Here's how the part is built. I have some questions about the finished solid (model axes, mm). Face numbers are marked on the shaded views. A direction names the side the tool comes from. Round coordinates to 2 decimals unless told otherwise and drop trailing zeros. Order: outer loops, then holes, each group sorted by start corner. A loop starts at its lowest first (then second) coordinate and runs counter-clockwise, first axis right, second up. Notation, with made-up numbers: M -14.5,71.5 L -4.5,71.5 A20 ccw -4.5,104.5 Z; hole C 68.25,-12 d3. An arc over 180 degrees is marked long. Answer as CSV lines item,"result". Start each with the question number.
```python
from build123d import *

# Parameters (mm, degrees)
F0_R     = 6.185827
F0_R_2   = 11.25
F1_DEPTH = 8.382


with BuildPart() as f1:
    # F0 (on Top) → F1 (new body)
    with BuildSketch(Plane.XY):
        with BuildLine():
            ThreePointArc((-10.795, 16.51), (-11.079307, 11.856451), (-11.927998, 7.272122))
            ThreePointArc((-11.927998, 7.272122), (-12.098375, 6.985), (-12.261842, 6.693888))
            ThreePointArc((-12.261842, 6.693888), (-15.807641, 3.666735), (-19.695579, 1.093744))
            Line((-19.695579, 1.093744), (-32.893807, -6.526256))
            ThreePointArc((-32.893807, -6.526256), (-35.852436, -10.382016), (-35.218068, -15.200517))
            Line((-35.218068, -15.200517), (-30.773068, -22.899483))
            ThreePointArc((-30.773068, -22.899483), (-26.917308, -25.858112), (-22.098807, -25.223744))
            Line((-22.098807, -25.223744), (-8.900579, -17.603744))
            ThreePointArc((-8.900579, -17.603744), (-4.728335, -15.523187), (-0.333844, -13.96601))
            ThreePointArc((-0.333844, -13.96601), (0, -13.97), (0.333844, -13.96601))
            ThreePointArc((0.333844, -13.96601), (4.728335, -15.523187), (8.900579, -17.603744))
            Line((8.900579, -17.603744), (22.098807, -25.223744))
            ThreePointArc((22.098807, -25.223744), (26.917308, -25.858112), (30.773068, -22.899483))
            Line((30.773068, -22.899483), (35.218068, -15.200517))
            ThreePointArc((35.218068, -15.200517), (35.852436, -10.382016), (32.893807, -6.526256))
            Line((32.893807, -6.526256), (19.695579, 1.093744))
            ThreePointArc((19.695579, 1.093744), (15.807641, 3.666735), (12.261842, 6.693888))
            ThreePointArc((12.261842, 6.693888), (12.098375, 6.985), (11.927998, 7.272122))
            ThreePointArc((11.927998, 7.272122), (11.079307, 11.856451), (10.795, 16.51))
            Line((10.795, 16.51), (10.795, 31.75))
            ThreePointArc((10.795, 31.75), (8.935128, 36.240128), (4.445, 38.1))
            Line((4.445, 38.1), (-4.445, 38.1))
            ThreePointArc((-4.445, 38.1), (-8.935128, 36.240128), (-10.795, 31.75))
            Line((-10.795, 31.75), (-10.795, 16.51))
        make_face()
        with Locations((-23.646824, -13.6525)):
            Circle(F0_R, mode=Mode.SUBTRACT)
        with Locations((23.646824, -13.6525)):
            Circle(F0_R, mode=Mode.SUBTRACT)
        Circle(F0_R_2, mode=Mode.SUBTRACT)
        with Locations((0, 27.305)):
            Circle(F0_R, mode=Mode.SUBTRACT)
    extrude(amount=F1_DEPTH)


solid = f1.part
```
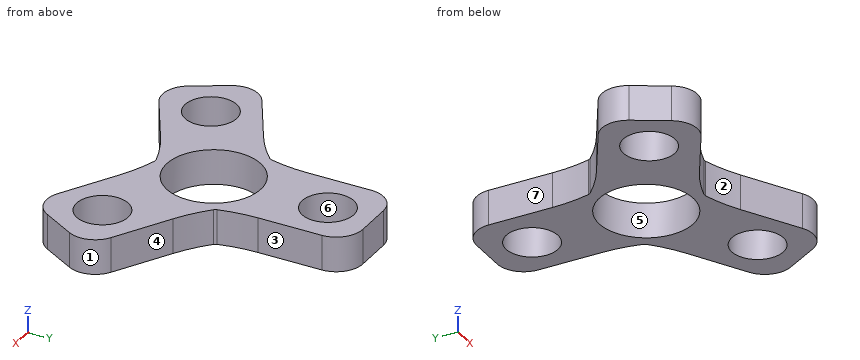
Item 1: If we section it at A-A on y = 0: Please give me the cut outline in (x, z).
Item 2: If we section it at C-C on x = -2.5: Please give me the cut outline in (y, z).
Item 3: If we section it at D-D on x = -29: Please give me the cut outline in (y, z), and give its area (3 significant figures).
Item 4: Which directions (+Z, -Z, +X, -X, +Y, -Y) give clear straight access to the entire face, cutting with the end or side of a thin tool? Please do the marked faces 1, 2 and 3.
Item 5: We'd pull the mould along Y, two halves only. Please class the marked faces 4, 5, 6 and 7: pulls with the +Y half, pulls with the -Y half, needs draft (parallel to the pull), parting line crosses it, or undercut.
Item 6: If I drill on line 1 along Y through (x, z) = (-3, 6); line 2 along X through (y, z) = (-8.5, 8.25); line 3 along X through (y, z) = (4.5, 5), over which ranges is the centre line in solid material (lowest first)?
Item 7: If we section it at B-B on z = 5.25: Count the separate pieces of the cut face and the enclosed holes in it, and give its area (3 significant figures).
Item 8: For P1, Ø4, axis at y = 21.5, z = 5, coming from the -X side (3 decimals); P2, Ø1.5, axis at x = 21, z = 2, coming from the -Y side; P3, Ø3, axis at y = 28, z = 4, coming from the +X side (3 decimals); P4, Ø18, axis at x = 0, y = 0, coming from the -Z side, each with a flat end and sliding along its axis, tell me the tip position at first contact or that it passes through.
Geometry says:
1,outline,"M -21.59,0 L -11.25,0 L -11.25,8.38 L -21.59,8.38 Z; M 11.25,0 L 21.59,0 L 21.59,8.38 L 11.25,8.38 Z"
2,outline,"M -14.66,0 L -10.97,0 L -10.97,8.38 L -14.66,8.38 Z; M 10.97,0 L 21.65,0 L 21.65,8.38 L 10.97,8.38 Z; M 32.96,0 L 38.1,0 L 38.1,8.38 L 32.96,8.38 Z"
3,outline,"M -24.87,0 L -16.75,0 L -16.75,8.38 L -24.87,8.38 Z; M -10.55,0 L -4.28,0 L -4.28,8.38 L -10.55,8.38 Z"
3,area,"121 mm²"
4,face 1,"+Z, -Z, +X"
4,face 2,"+Z, -Z, -Y"
4,face 3,"+Z, -Z, +X, +Y"
5,face 4,"pulls with the +Y half"
5,face 5,"undercut"
5,face 6,"undercut"
5,face 7,"needs draft"
6,line 1,"-14.84 to -10.84, 10.84 to 21.9, 32.71 to 38.1"
6,line 2,"-35 to -27.07, -20.22 to -7.37, 7.37 to 20.22, 27.07 to 35"
6,line 3,"-14.74 to -10.31, 10.31 to 14.74"
7,separate pieces,"1"
7,enclosed holes,"4"
7,area,"1,480 mm²"
8,P1,"x = -10.795"
8,P2,"y = -25.02"
8,P3,"x = 10.795"
8,P4,"through"
